from build123d import *

# Parameters (mm, degrees)
SKETCH1_W           = 12.7
SKETCH1_H           = 31.75
SKETCH1_R           = 3.175
BOSS_EXTRUDE2_DEPTH = 3.175
SKETCH2_W           = 12.7
SKETCH2_H           = 3.175
BOSS_EXTRUDE4_DEPTH = 22.225
SKETCH3_R           = 3.175
BOSS_EXTRUDE5_DEPTH = 3.175


with BuildPart() as part:
    # Sketch1 → Boss-Extrude2 (new body)
    with BuildSketch(Plane(origin=(0, 0, 0), x_dir=(1, 0, 0), z_dir=(0, 1, 0))):
        with Locations((6.35, 15.875)):
            Rectangle(SKETCH1_W, SKETCH1_H)
        with Locations((4.826, 15.875)):
            Circle(SKETCH1_R, mode=Mode.SUBTRACT)
    extrude(amount=BOSS_EXTRUDE2_DEPTH)

    # Sketch2 → Boss-Extrude4 (add)
    with BuildSketch(Plane(origin=(0, 3.175, 0), x_dir=(1, 0, 0), z_dir=(0, 1, 0))):
        Polygon((12.7, 31.75), (0, 31.75), (0, 28.575), (11.684, 28.575), (12.7, 28.575), align=None)
        with Locations((6.35, 1.5875)):
            Rectangle(SKETCH2_W, SKETCH2_H)
    extrude(amount=BOSS_EXTRUDE4_DEPTH)

    # Sketch3 → Boss-Extrude5 (add)
    with BuildSketch(Plane(origin=(0, 25.4, 0), x_dir=(1, 0, 0), z_dir=(0, 1, 0))):
        Polygon((12.7, 28.575), (12.7, 31.75), (0, 31.75), (0, 28.575), (0, 3.175), (0, 0), (12.7, 0), (12.7, 3.175), align=None)
        with Locations((4.826, 15.875)):
            Circle(SKETCH3_R, mode=Mode.SUBTRACT)
    extrude(amount=BOSS_EXTRUDE5_DEPTH)


solid = part.part
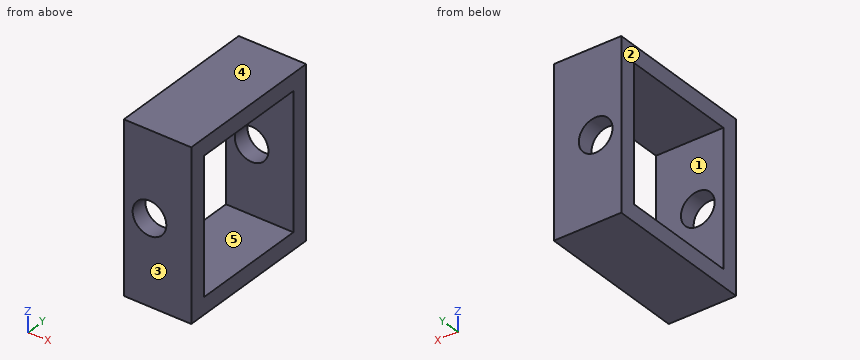
Read the model definition and answer for the solid it produces. Units are mm, in the model's axes. Face numbers are marked on the shaded views. A direction names the side the tool comes from. Coordinates: 2 decimals unless noted, no trailing zeros. Loops run counter-clockwise (first coordinate to the right, second up) from the corner with the lowest first, then second, coordinate; pieces in that order, holes last.
Q1. The part is cut by section D-D on z = -14. Write down the section's boundary in (x, y) (3 decimals).
Q2. The part is cut by section A-A on z = -7. Write down the section's boundary in (x, y) (3 decimals).
Q3. The part is cut by section B-B on x = 9. Write down the section's boundary in (y, z) (3 decimals), and give its area (3 significant figures).
Q4. The mould has two halves that part along Y. Classify the marked faces 3, 4 and 5: +Y half, -Y half, draft (parallel to the pull), parting line (faces both ways), or undercut.
Q5. Consider probe 1 along Y at (x, z) = (9.5, -23) (3 decimals); probe 2 along Z at (x, y) = (1, 14.5) (3 decimals). Determine where each line is inside the solid, lowest interval first.
Q6. Which of the six approach directions +Z, -Z, +X, -X, +Y, -Y give full straight-line access (tool end or side, diameter ignored) to the marked faces 1 and 2?
Q7. The part is cut by section C-C on y = 21.25. Write down the section's boundary in (x, z) (3 decimals), and give its area (3 significant figures).
Results below:
1. outline: (0, 0) - (2.264, 0) - (2.264, 3.175) - (0, 3.175) - close; (0, 25.4) - (2.264, 25.4) - (2.264, 28.575) - (0, 28.575) - close; (7.388, 0) - (12.7, 0) - (12.7, 3.175) - (7.388, 3.175) - close; (7.388, 25.4) - (12.7, 25.4) - (12.7, 28.575) - (7.388, 28.575) - close
2. outline: (0, 0) - (12.7, 0) - (12.7, 3.175) - (0, 3.175) - close; (0, 25.4) - (12.7, 25.4) - (12.7, 28.575) - (0, 28.575) - close
3. outline: (0, -31.75) - (28.575, -31.75) - (28.575, 0) - (0, 0) - close; hole (3.175, -28.575) - (25.4, -28.575) - (25.4, -3.175) - (3.175, -3.175) - close
3. area: 343 mm2
4. face 3: -Y half
4. face 4: draft
4. face 5: undercut
5. probe 1: y = 0 to 3.175, 25.4 to 28.575
5. probe 2: z = -31.75 to -28.575, -3.175 to 0
6. face 1: +X, -X
6. face 2: +Z, -Z, -X, +Y, -Y
7. outline: (0, -31.75) - (12.7, -31.75) - (12.7, -28.575) - (0, -28.575) - close; (0, -3.175) - (12.7, -3.175) - (12.7, 0) - (0, 0) - close
7. area: 80.6 mm2
